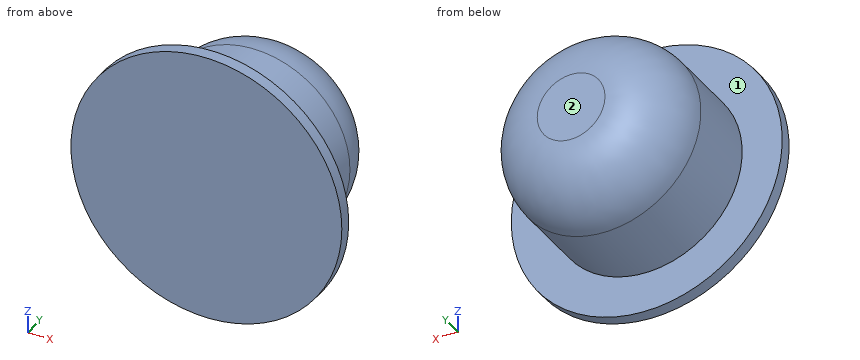
```python
from build123d import *

# Parameters (mm, degrees)
F0_R     = 7.75
F1_DEPTH = 12
F0_R_2   = 11
F2_DEPTH = 1
F3_R     = 5


with BuildPart() as f1:
    # F0 (on Front) → F1 (new body)
    with BuildSketch(Plane.XZ):
        Circle(F0_R)
    extrude(amount=-F1_DEPTH)

    # F0 (on Front) → F2 (join)
    with BuildSketch(Plane.XZ):
        Circle(F0_R_2)
        Circle(F0_R, mode=Mode.SUBTRACT)
    extrude(amount=-F2_DEPTH)

    # F3
    f3_edges = [f1.edges().sort_by_distance(p)[0] for p in [
        (-7.75, 12, 0),
    ]]
    fillet(f3_edges, radius=F3_R)


solid = f1.part
```
The listing builds one solid part. Answer for the finished solid, in the listing's coordinates (mm). Face numbers are marked on the shaded views. A direction names the side the tool comes from. Coordinates: 2 decimals unless noted, no trailing zeros. Write each loop counter-clockwise with the first axis right and the second up, starting at its lowest first coordinate (ties: lowest second). Pieces come first, ordered by that corner, then holes. Notation, with made-up numbers: M 25.25,23.5 L 61.25,23.5 A30 ccw 61.25,50.5 Z; hole C -18.75,-19.75 d3. An arc over 180 degrees is marked long. Use a Markdown table: item, result. Add a question column.
1. Section B-B (z = 9) is taken. Give the vertices of the cut face in (x, y).
2. Straight lines are drawn through the part: line 1 along X through (y, z) = (2, -0.25); line 2 along Y through (x, z) = (3.5, 8.75); line 3 along X through (y, z) = (10, -4.75). For each, find the intervals that lie inside material, in ascending order. Write a range as [from, to].
3. Section C-C (x = 9.25) is taken. Give the vertices of the cut face in (y, z).
4. Which of the six approach directions +Z, -Z, +X, -X, +Y, -Y give full straight-line access (tool end or side, diameter ignored) to the marked faces 1 and 2?
5. Given P1, Ø6, axis at x = -2.5, y = 6, coming from the -Z side; P2, Ø3, axis at x = 7.5, y = 7, coming from the -Z side; P3, Ø2, axis at y = 6.5, z = -5, coming from the +X side, each flat-ended and moving along its own axis, determine where each tip first touches the part or whether it passes through.
6. Section A-A (y = 4.75) is taken. Give the vertices of the cut face in (x, z).
Data:
| question | item | result |
|---|---|---|
| 1 | outline | M -6.32,0 L 6.32,0 L 6.32,1 L -6.32,1 Z |
| 2 | line 1 | x = [-7.75, 7.75] |
| 2 | line 2 | y = [0, 1] |
| 2 | line 3 | x = [-4.8, 4.8] |
| 3 | outline | M 0,-5.95 L 1,-5.95 L 1,5.95 L 0,5.95 Z |
| 4 | face 1 | +Y |
| 4 | face 2 | +Z, -Z, +X, -X, +Y |
| 5 | P1 | stops at z = -7.75 |
| 5 | P2 | stops at z = -4.91 |
| 5 | P3 | stops at x = 6.64 |
| 6 | outline | C 0,0 d15.5 |
